Geometry check sheet. Reference: drawing and pictorial views, mm from the part's lowest x, y, z. Give positions to 0.01 mm unless a question says otherwise; leave off trailing zeros. Order: outer loops, then holes, each group sorted by start corner. A loop starts at its lowest first (then second) coordinate and runs counter-clockwise, first axis right, second up.
Item 1: Gauge pin test, flat ends, axial feed: P1, Ø10, axis at x = 31, y = 41, coming from the -Z side; P2, Ø2, axis at y = 16, z = 6, coming from the +X side; P3, Ø2, axis at x = 44, z = 5.5, coming from the +Y side; P4, Ø5, axis at x = 16, z = 6, coming from the -Y side. Record the tip position at first contact, or that the pin passes through.
Item 2: Release check for a two-part mould opening along X. For the marked faces 1, 2 and 3 record: released by +X, released by -X, zero draft, split by the parting line, or undercut.
Item 3: Sectioned sample at A-A on x = 25. Record the boundary of the cut face in (y, z).
Item 4: Material ranges on line 1 along Y through (x, z) = (25, 5.5); line 2 along X through (y, z) = (29.5, 1); line 3 along X through (y, z) = (29, 1.5), recorded low to high.
Item 5: Sectioned sample at D-D on z = 5.5. Record the boundary of the cut face in (x, y).
Item 6: Sectioned sample at B-B on y = 39.5. Record the boundary of the cut face in (x, z) (1 decimal), and give its area (3 significant figures).
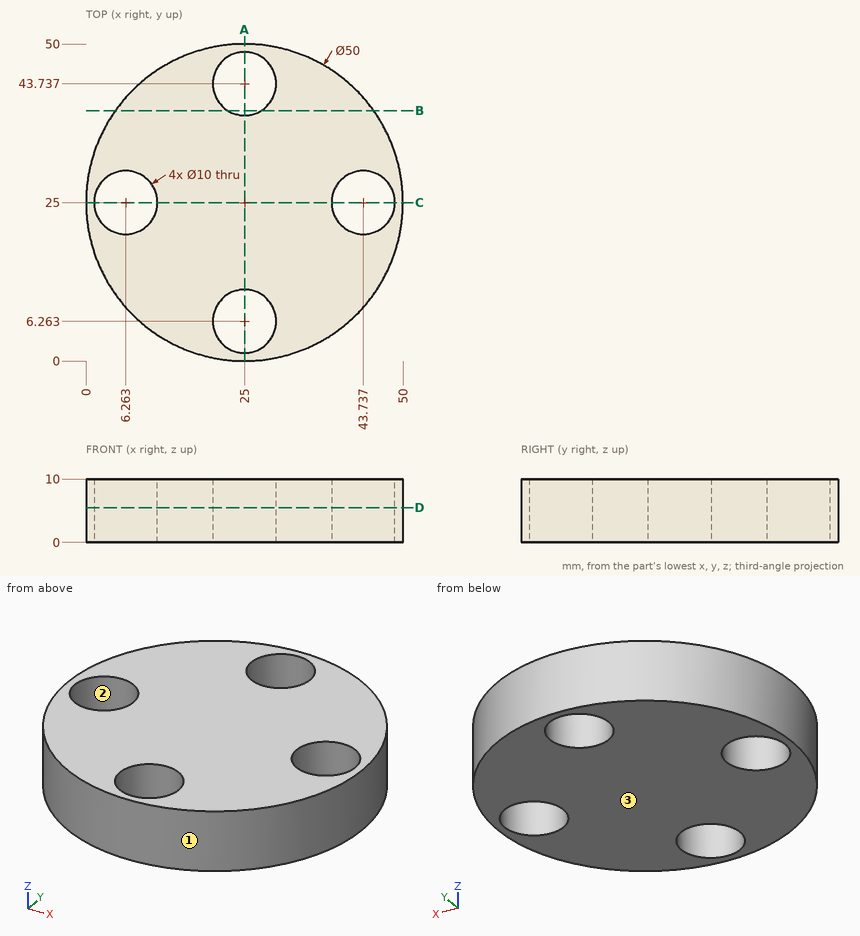
Report:
1. P1: stops at z = 0
1. P2: stops at x = 48.69
1. P3: stops at y = 42.35
1. P4: stops at y = 0.86
2. face 1: split by the parting line
2. face 2: undercut
2. face 3: zero draft
3. outline: (0, 0) - (1.26, 0) - (1.26, 10) - (0, 10) - close; (11.26, 0) - (38.74, 0) - (38.74, 10) - (11.26, 10) - close; (48.74, 0) - (50, 0) - (50, 10) - (48.74, 10) - close
4. line 1: y = 0 to 1.26, 11.26 to 38.74, 48.74 to 50
4. line 2: x = 0.41 to 4.08, 8.44 to 41.56, 45.92 to 49.59
4. line 3: x = 0.32 to 3.26, 9.26 to 40.74, 46.74 to 49.68
5. outline: circle Ø50 at (25, 25); hole circle Ø10 at (6.26, 25); hole circle Ø10 at (25, 6.26); hole circle Ø10 at (25, 43.74); hole circle Ø10 at (43.74, 25)
6. outline: (4.6, 0) - (22.3, 0) - (22.3, 10) - (4.6, 10) - close; (27.7, 0) - (45.4, 0) - (45.4, 10) - (27.7, 10) - close
6. area: 354 mm2
